Geometry: final body of the model. Coordinates: model frame, mm. Give positions to 0.01 mm unless a question says otherwise; leave off trailing zeros. Write each loop counter-clockwise with the first axis right and the second up, starting at its lowest first coordinate (ties: lowest second). Pieces come first, ordered by that corner, then holes. Notation, with made-up numbers: (76.5, -5) - (89.5, -5) arc R31 ccw to (89.5, 28) - close; hole circle Ø1 at (-24.75, 85). An arc over 180 degrees is marked (long way). Use CSV: the item, a comma, the result in double quotes. Start each with the question number.
(1) Section A-A on z = -18. Output: boundary loops of the cut face in (x, y), and give its area (3 significant figures).
(2) Section D-D on z = -10.5. Output: boundary loops of the cut face in (x, y).
(3) Section C-C on y = -3.5. Output: boundary loops of the cut face in (x, z), and give its area (3 significant figures).
(4) Line query: probe 1 along Z at (x, y) = (20, 2.8); probe 2 along X at (y, z) = (-1.8, -18); probe 3 along X at (y, z) = (4.55, -18). Output: solid intervals per line, ascending. Write a range as [from, to].
(5) Section B-B on x = 20. Output: boundary loops of the cut face in (y, z), and give its area (3 significant figures).
(6) First-contact query: pin 1 Ø5 at (x, z) = (-20, -18) entering from +Y; pin 2 Ø1 at (x, y) = (2.5, 2) entering from +Z. Flat tips, straight axial feed; report the tip coordinate or a pass-through.
from build123d import *

# Parameters (mm, degrees)
BOSS_EXTRUDE1_DEPTH = 36
SKETCH2_R           = 4
CUT_EXTRUDE1_DEPTH  = 7
SKETCH3_R           = 4
CUT_EXTRUDE2_DEPTH  = 7


with BuildPart() as part:
    # Sketch1 → Boss-Extrude1 (new body)
    with BuildSketch(Plane.XY):
        with BuildLine():
            Line((10, 6), (37, 6))
            Line((37, 6), (37, -6))
            Line((37, -6), (-37, -6))
            Line((-37, -6), (-37, 6))
            Line((-37, 6), (-10, 6))
            ThreePointArc((-10, 6), (0, 2.489995997), (10, 6))
        make_face()
    extrude(amount=-BOSS_EXTRUDE1_DEPTH)

    # Sketch2 → Cut-Extrude1 (cut, through all)
    with BuildSketch(Plane(origin=(0, 0, 0), x_dir=(1, 0, 0), z_dir=(0, 1, 0))):
        with Locations((-20, 18)):
            Circle(SKETCH2_R)
        with Locations((20, 18)):
            Circle(SKETCH2_R)
    extrude(amount=CUT_EXTRUDE1_DEPTH, mode=Mode.SUBTRACT)

    # Sketch3 → Cut-Extrude2 (cut, through all)
    with BuildSketch(Plane(origin=(0, 0, 0), x_dir=(1, 0, 0), z_dir=(0, 1, 0))):
        with Locations((-20, 18)):
            Circle(SKETCH3_R)
        with Locations((20, 18)):
            Circle(SKETCH3_R)
    extrude(amount=-CUT_EXTRUDE2_DEPTH, mode=Mode.SUBTRACT)


solid = part.part
Check values:
1,outline,"(-37, -6) - (-24, -6) - (-24, 6) - (-37, 6) - close; (-16, -6) - (16, -6) - (16, 6) - (10, 6) arc R16 cw to (-10, 6) - (-16, 6) - close; (24, -6) - (37, -6) - (37, 6) - (24, 6) - close"
1,area,"648 mm²"
2,outline,"(-37, -6) - (37, -6) - (37, 6) - (10, 6) arc R16 cw to (-10, 6) - (-37, 6) - close"
3,outline,"(-37, -36) - (37, -36) - (37, 0) - (-37, 0) - close; hole circle Ø8 at (-20, -18); hole circle Ø8 at (20, -18)"
3,area,"2,560 mm²"
4,probe 1,"z = [-36, -22], [-14, 0]"
4,probe 2,"x = [-37, -24], [-16, 16], [24, 37]"
4,probe 3,"x = [-37, -24], [-16, -7.85], [7.85, 16], [24, 37]"
5,outline,"(-6, -36) - (6, -36) - (6, -22) - (-6, -22) - close; (-6, -14) - (6, -14) - (6, 0) - (-6, 0) - close"
5,area,"336 mm²"
6,pin 1,"passes through"
6,pin 2,"stops at z = 0"
